Autodesk Inventor part; units mm, degrees
ref_plane "YZ Plane" through (0, 0, 0) normal (1, 0, 0) x (0, 1, 0)
ref_plane "XZ Plane" through (0, 0, 0) normal (0, 1, 0) x (-1, 0, 0)
ref_plane "XY Plane" through (0, 0, 0) normal (0, 0, 1) x (1, 0, 0)
sketch "Sketch_1" plane through (0, 0, 0) normal (0, 0, 1) x (1, 0, 0)
  line L0 (9, 0) -> (0, 0)
  line L1 (0, 11.725) -> (0.3, 11.425)
  line L2 (0.3, 11.425) -> (1.7844, 11.425)
  arc A0 (5.097, 13.09) -> (1.7844, 11.425) centre (4.5, 10.15) ccw
  line L3 (5.097, 13.09) -> (8.8, 13.09)
  arc A1 (8.8, 13.09) -> (9, 13.29) centre (8.8, 13.29) ccw
  line L4 (9, 13.29) -> (9, 14.7)
  arc A2 (9, 14.7) -> (8.7, 15) centre (8.7, 14.7) ccw
  line L5 (8.7, 15) -> (0.6, 15)
  arc A3 (0.6, 15) -> (0, 14.4) centre (0.6, 14.4) ccw
  line L6 (0, 14.4) -> (0, 11.725)
revolve "Revolution1" add sketch "Sketch_1" angle 360 about axis through (9, 0, 0) along (1, 0, 0)
properties part number "SKF_7200 BECBP_PART2"
Verification items for the finished model (mm, model axes). Give positions to 0.01 mm unless a question says otherwise; leave off trailing zeros. Loops run counter-clockwise (first coordinate to the right, second up) from the corner with the lowest first, then second, coordinate; pieces in that order, holes last.
1) Sectioned sample at C-C, the plane x = 7.25. Enter the section's corners in (y, z), then the cut area to 3 significant figures.
2) Draft check along Y on faces 1 (the flat face through (9, -11, -8)), 2 (the cylindrical face through (4.593, -14.985, -0.66)), 3 (the cylindrical face through (6.97, -2.84, -12.78)). Enter one of: pulls with the +Y half, pulls with the -Y half, needs draft (parallel to the pull), parting line crosses it, or undercut.
3) Sectioned sample at A-A, the plane y = 0. Enter the section's corners in (x, z) (3 decimals), then the cut area to 3 significant figures.
4) Depth check by flat-ended pin: pin 1 Ø6 at (y, z) = (0, -7) entering from +X; pin 2 Ø4 at (x, y) = (4.5, 5) entering from -Z; pin 3 Ø8 at (y, z) = (3, -10.5) entering from +X. Enter the tip coordinate at first touch or a pass-through.
5) Thickness scan on line 1 along Z through (x, y) = (7.4, 0); line 2 along Z through (x, y) = (1.35, 0) (3 decimals); line 3 along Y through (x, z) = (3.5, 10.5). Record the ranges inside material, lowest first.
6) Sectioned sample at D-D, the plane x = 3.75. Enter the section's corners in (y, z), then the cut area to 3 significant figures.
Answers:
1. outline: circle Ø30 at (0, 0); hole circle Ø26.18 at (0, 0)
1. area: 169 mm2
2. face 1: needs draft
2. face 2: parting line crosses it
2. face 3: undercut
3. outline: (0, -14.4) arc R0.6 ccw to (0.6, -15) - (8.7, -15) arc R0.3 ccw to (9, -14.7) - (9, -13.29) arc R0.2 ccw to (8.8, -13.09) - (5.097, -13.09) arc R3 cw to (1.784, -11.425) - (0.3, -11.425) - (0, -11.725) - close; (0, 11.725) - (0.3, 11.425) - (1.784, 11.425) arc R3 cw to (5.097, 13.09) - (8.8, 13.09) arc R0.2 ccw to (9, 13.29) - (9, 14.7) arc R0.3 ccw to (8.7, 15) - (0.6, 15) arc R0.6 ccw to (0, 14.4) - close
3. area: 42.3 mm2
4. pin 1: passes through
4. pin 2: stops at z = -14.7
4. pin 3: stops at x = 9
5. line 1: z = -15 to -13.09, 13.09 to 15
5. line 2: z = -15 to -11.425, 11.425 to 15
5. line 3: y = -10.71 to -7.63, 7.63 to 10.71
6. outline: circle Ø30 at (0, 0); hole circle Ø26.11 at (0, 0)
6. area: 171 mm2
